Source: CAD feature listing. Evaluate the final solid. Frame: model axes, mm. Face numbers are marked on the shaded views. A direction names the side the tool comes from. Give positions to 0.01 mm unless a question says otherwise; leave off trailing zeros. Order: outer loops, then holes, each group sorted by start corner. A loop starts at its lowest first (then second) coordinate and runs counter-clockwise, first axis right, second up.
from build123d import *

# Parameters (mm, degrees)
SKIZZE5_W                            = 0.8
SKIZZE5_H                            = 4.5
SKIZZE7_R                            = 1.25
SCHNITT_LINEAR_AUSTRAGEN2_DEPTH      = 5.50000011
SCHNITT_LINEAR_AUSTRAGEN2_DEPTH_BACK = 5.5000001


with BuildPart() as part:
    # Skizze1 → Rotation1 (revolve)
    with BuildSketch(Plane.XY):
        Polygon((0, 4.5), (0, 2), (14, 2), (15.201721238, 0), (21, 0), (21, 3), (15, 3), (15, 4.5), align=None)
    revolve(axis=Axis((0, 0, 0), (1, 0, 0)))

    # Skizze5 → M2 Gewindebohrung1 (revolve, cut)
    with BuildSketch(Plane.YZ.offset(7)):
        with Locations((0.4, 2.25)):
            Rectangle(SKIZZE5_W, SKIZZE5_H)
    revolve(axis=Axis((7, 0, -6.35), (0, 0, 1)), mode=Mode.SUBTRACT)

    # Skizze7 → Schnitt-Linear austragen2 (cut, two sides)
    with BuildSketch(Plane.XY) as schnitt_linear_austragen2_sk:
        with Locations((12, 0)):
            Circle(SKIZZE7_R)
    extrude(amount=SCHNITT_LINEAR_AUSTRAGEN2_DEPTH, mode=Mode.SUBTRACT)
    extrude(schnitt_linear_austragen2_sk.sketch, amount=-SCHNITT_LINEAR_AUSTRAGEN2_DEPTH_BACK, mode=Mode.SUBTRACT)


solid = part.part
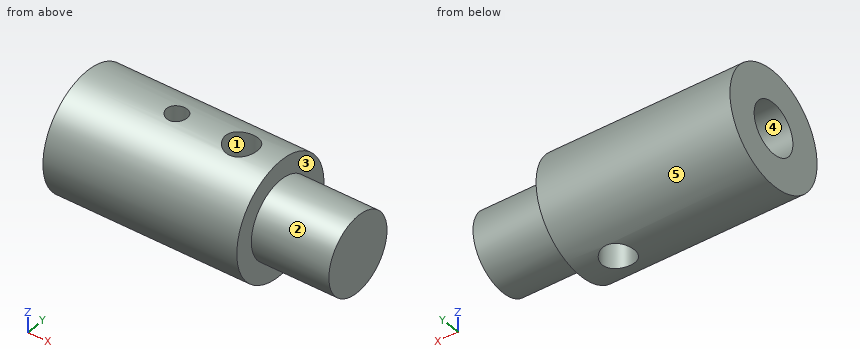
1) Section query C-C on x = 2.5. Output: boundary loops of the cut face in (y, z), and give its area (3 significant figures).
Checks:
outline: circle Ø9 at (0, 0); hole circle Ø4 at (0, 0)
area: 51.1 mm2
2) Section query B-B on z = -2.5. Output: boundary loops of the cut face in (x, y).
Checks:
outline: (0, -3.74) - (15, -3.74) - (15, -1.66) - (21, -1.66) - (21, 1.66) - (15, 1.66) - (15, 3.74) - (0, 3.74) - close; hole circle Ø2.5 at (12, 0)
3) Section query D-D on y = -1. State how many separate pieces and enclosed holes the cut face has, and give its area (3 significant figures).
Checks:
separate pieces: 3
enclosed holes: 0
area: 108 mm2
4) Pull-direction query (X, two-part tool) for the marked faces 1, 2 and 3; classes: +X half, -X half, draft (parallel to the pull), parting line (faces both ways), or undercut.
Checks:
face 1: undercut
face 2: draft
face 3: +X half
5) Reachability of the marked faces 4 and 5 from +Z, -Z, +X, -X, +Y, -Y: full face, straight path, thin tool, end or side. Return the list, or none.
Checks:
face 4: -X
face 5: +X, -X
6) Ray query, L1, parallel to X at y = 0, z = 2.4; L2, parallel to X at y = -0.5, z = 3.75; L3, parallel to Y at x = 1.5, z = 1.75. Return the intervals inside material, ascending.
Checks:
L1: x = 0 to 6.2, 7.8 to 10.75, 13.25 to 21
L2: x = 0 to 6.38, 7.62 to 10.85, 13.15 to 15
L3: y = -4.15 to -0.97, 0.97 to 4.15
7) First-contact query: pin 1 Ø1 at (x, z) = (8.5, 3) entering from -Y; pin 2 Ø3 at (x, y) = (17.5, 0) entering from +Z; pin 3 Ø4 at (x, y) = (4.5, -3.5) entering from -Z; pin 4 Ø1.5 at (x, y) = (12, 0) entering from +Z. Flat tips, straight axial feed; report the tip coordinate or a pass-through.
Checks:
pin 1: stops at y = -3.74
pin 2: stops at z = 3
pin 3: stops at z = -4.24
pin 4: passes through
8) Section query A-A on x = 12.75. Output: boundary loops of the cut face in (y, z).
Checks:
outline: (-1, -4.39) - (-1, -1.73) arc R2 cw to (-1, 1.73) - (-1, 4.39) arc R4.5 ccw to start; (1, -4.39) arc R4.5 ccw to (1, 4.39) - (1, 1.73) arc R2 cw to (1, -1.73) - close
